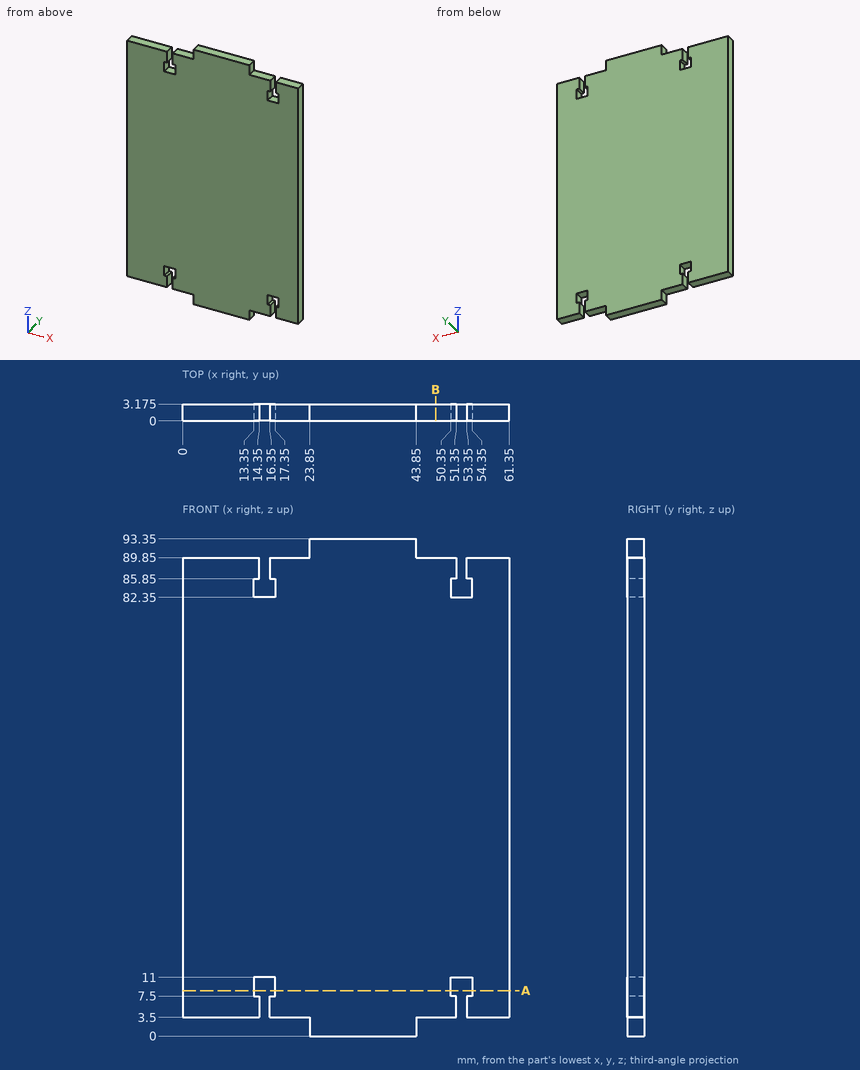
Print and shaded views of the part. All mm, measured from the part's lowest x, y and z. Give positions to 0.01 mm unless a question says otherwise; leave off trailing zeros. Loops run counter-clockwise (first coordinate to the right, second up) from the corner with the lowest first, then second, coordinate; pieces in that order, holes last. Notation, with made-up numbers: (22, 38.5) - (81, 38.5) arc R23 cw to (81, 46.5) - close; hole circle Ø8 at (63.25, -37.75). An arc over 180 degrees is marked (long way). Use a Markdown table: item, result.
(1) Band-saw the part on A-A (z = 8.5). Give the cut face in (x, y) (3 decimals).
Taken from the geometry:
| item | result |
|---|---|
| outline | (0, 0) - (13.35, 0) - (13.35, 3.175) - (0, 3.175) - close; (17.35, 0) - (50.35, 0) - (50.35, 3.175) - (17.35, 3.175) - close; (54.35, 0) - (61.35, 0) - (61.35, 3.175) - (54.35, 3.175) - close |
(2) Band-saw the part on B-B (x = 47.5). Give the cut face in (y, z) (3 decimals), and give its area (3 significant figures).
Taken from the geometry:
| item | result |
|---|---|
| outline | (0, 3.5) - (3.175, 3.5) - (3.175, 89.85) - (0, 89.85) - close |
| area | 274 mm2 |
(3) Wall check: line 1 along X through (y, z) = (1.8, 82.5); line 2 along X through (y, z) = (0.4, 88); line 3 along Z through (x, y) = (51, 0.65). Give the ranges that are in metal, low to high.
Taken from the geometry:
| item | result |
|---|---|
| line 1 | 0 to 13.35, 17.35 to 50.35, 54.35 to 61.35 |
| line 2 | 0 to 14.35, 16.35 to 51.35, 53.35 to 61.35 |
| line 3 | 3.5 to 7.5, 11 to 82.35, 85.85 to 89.85 |
(4) Drop flat-ended pins along their axis: pin 1 Ø1.6 at (x, y) = (20, 2) entering from -Z; pin 2 Ø1 at (y, z) = (1, 1.5) entering from +X; pin 3 Ø1 at (y, z) = (1, 87.5) entering from -X. Give the stop position or say it passes through.
Taken from the geometry:
| item | result |
|---|---|
| pin 1 | z = 3.5 |
| pin 2 | x = 43.85 |
| pin 3 | x = 0 |
